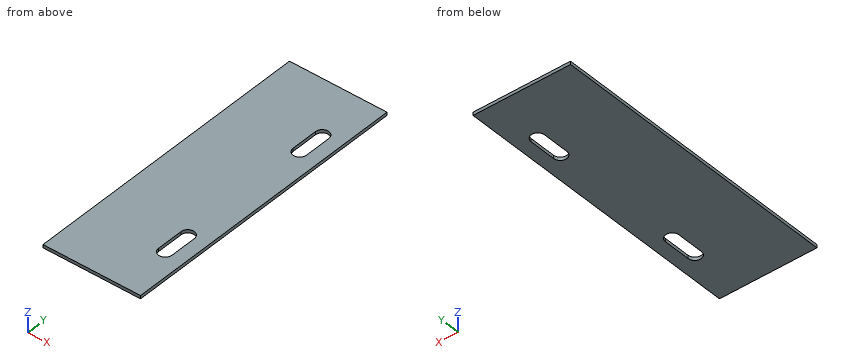
Autodesk Inventor part; units mm, degrees
ref_plane "YZ Plane" through (0, 0, 0) normal (1, 0, 0) x (0, 1, 0)
ref_plane "XZ Plane" through (0, 0, 0) normal (0, 1, 0) x (-1, 0, 0)
ref_plane "XY Plane" through (0, 0, 0) normal (0, 0, 1) x (1, 0, 0)
sketch "Skizze1" plane through (0, 0, 0) normal (0, 0, 1) x (1, 0, 0)
  line L0 (0, 0) -> (36.5, 0)
  line L1 (36.5, 0) -> (36.5, 110)
  line L2 (36.5, 110) -> (0, 110)
  line L3 (0, 110) -> (0, 91.5)
  line L4 (0, 86.5) -> (0, 91.5)
  line L5 (0, 18.5) -> (0, 23.5)
  line L6 (0, 23.5) -> (0, 18.5) construction
  line L7 (0, 18.5) -> (0, 0)
  line L8 (0, 86.5) -> (0, 23.5)
  line L9 (0, 91.5) -> (0, 86.5) construction
  line L10 (31.5, 90) -> (26.5, 90) construction
  line L11 (26.5, 90) -> (26.5, 80)
  line L12 (26.5, 80) -> (31.5, 80) construction
  line L13 (31.5, 80) -> (31.5, 90)
  line L14 (31.5, 30) -> (26.5, 30) construction
  line L15 (26.5, 30) -> (26.5, 20)
  line L16 (26.5, 20) -> (31.5, 20) construction
  line L17 (31.5, 20) -> (31.5, 30)
  line L18 (29, 80) -> (29, 30) construction
  line L19 (36.5, 55) -> (0, 55) construction
  arc A0 (31.5, 90) -> (26.5, 90) centre (29, 90) ccw
  arc A1 (26.5, 80) -> (31.5, 80) centre (29, 80) ccw
  arc A2 (31.5, 30) -> (26.5, 30) centre (29, 30) ccw
  arc A3 (26.5, 20) -> (31.5, 20) centre (29, 20) ccw
  point P0 (29, 55)
  dimension "d0" = 36.5
  dimension "d1" = 110
  dimension "d10" = 10
  dimension "d11" = 10
  dimension "d12" = 5
  dimension "d13" = 5
  dimension "d15" = 20
extrude "Extrusion2" add sketch "Skizze1" along normal blind 1.2
properties part number "bett_V2_deckplatte_klappe" material "Holz (Walnuss)"
Work out the finished part from the listing and answer in its coordinate system (mm). Give positions to 0.01 mm unless a question says otherwise; leave off trailing zeros. Loops run counter-clockwise (first coordinate to the right, second up) from the corner with the lowest first, then second, coordinate; pieces in that order, holes last. Notation, with made-up numbers: (80.5, -8) - (139.5, -8) arc R27 cw to (139.5, 15) - close; hole circle Ø4 at (9, 40). An arc over 180 degrees is marked (long way). Answer in a Markdown table with one row per item.
(1) Consider L1, parallel to X at y = 23, z = 0.65; L2, parallel to Y at x = 30, z = 0.45. Determine where each line is inside the solid, lowest interval first. Write a range as [from, to].
Results list:
| item | result |
|---|---|
| L1 | x = [0, 26.5], [31.5, 36.5] |
| L2 | y = [0, 17.71], [32.29, 77.71], [92.29, 110] |
(2) Section A-A (x = 29) is taken. Give the vertices of the cut face in (y, z), and give its area (3 significant figures).
Results list:
| item | result |
|---|---|
| outline | (0, 0) - (17.5, 0) - (17.5, 1.2) - (0, 1.2) - close; (32.5, 0) - (77.5, 0) - (77.5, 1.2) - (32.5, 1.2) - close; (92.5, 0) - (110, 0) - (110, 1.2) - (92.5, 1.2) - close |
| area | 96.0 mm² |
(3) Section B-B (z = 0.6) is taken. Give the vertices of the cut face in (x, y), and give its area (3 significant figures).
Results list:
| item | result |
|---|---|
| outline | (0, 0) - (36.5, 0) - (36.5, 110) - (0, 110) - close; hole (26.5, 20) arc R2.5 ccw to (31.5, 20) - (31.5, 30) arc R2.5 ccw to (26.5, 30) - close; hole (26.5, 80) arc R2.5 ccw to (31.5, 80) - (31.5, 90) arc R2.5 ccw to (26.5, 90) - close |
| area | 3,880 mm² |
